Check sheet for the modelled part. Datum: model origin and axes. Units: mm. A direction names the side the tool comes from. Round coordinates to 2 decimals unless told otherwise and drop trailing zeros. Order: outer loops, then holes, each group sorted by start corner. A loop starts at its lowest first (then second) coordinate and runs counter-clockwise, first axis right, second up. Notation, with made-up numbers: (-15.5, 86.5) -> (-3.5, 86.5) arc R32 cw to (-3.5, 122.5) -> close; hole circle Ø7 at (87, 38.5). An arc over 180 degrees is marked (long way). Answer in a Markdown table with one row per item. Add a question column.
1. Material ranges on L1, parallel to X at y = 1.4, z = -2.55; L2, parallel to X at y = 2.25, z = 22.5; L3, parallel to X at y = 4.25, z = 13, recorded low to high. Write a range as from..to.
2. Draft check along Y on faces 5 (the cylindrical face through (3.55, 3.4, -2.97)), 6 (the conical face through (9.104, 5.907, 0.588)), 7 (the flat face through (9, 1.4, 2)). Enter one of: +Y half, -Y half, draft (parallel to the pull), parting line (faces both ways), or undercut.
3. Access from +Z, -Z, +X, -X, +Y, -Y to the whole of each face (thin tool, end or side, straight path). Record for faces 1 (the flat face through (16, 1.4, 17)), 2 (the flat face through (-3, 3, 4)), 3 (the cylindrical face through (-0.41, 4.9, 10.43)), 4 (the flat face through (3.9, 2.4, -1)).
4. Sectioned sample at C-C, the plane x = 3. Record the boundary of the cut face in (y, z).
5. Sectioned sample at D-D, the plane x = -2. Record the boundary of the cut face in (y, z), then the cut area to 3 significant figures.
6. Sectioned sample at B-B, the plane y = 4.75. Record the boundary of the cut face in (x, z).
7. Sectioned sample at A-A, the plane z = 11.5. Record the boundary of the cut face in (x, y).
8. Depth check by flat-ended pin: P1, Ø4.5, axis at x = 9, z = 0.26, coming from the +Y side; P2, Ø5, axis at x = 3.5, z = 23, coming from the -Y side; P3, Ø1.3, axis at x = 7.5, y = 4.5, coming from the -Z side; P4, Ø4, axis at y = 6, z = 10, coming from the -X side. Enter the tip coordinate at first touch or a pass-through.
Autodesk Inventor part; units mm, degrees
ref_plane "YZ Plane" through (0, 0, 0) normal (1, 0, 0) x (0, 1, 0)
ref_plane "XZ Plane" through (0, 0, 0) normal (0, 1, 0) x (-1, 0, 0)
ref_plane "XY Plane" through (0, 0, 0) normal (0, 0, 1) x (1, 0, 0)
sketch "Skizze1" plane through (0, 0, 0) normal (0, 1, 0) x (-1, 0, 0)
  line L0 (0, 0) -> (-18, 0)
  line L1 (-18, 0) -> (-18, 28)
  line L2 (-18, 28) -> (0, 28)
  line L3 (0, 28) -> (0, 0)
  dimension "d0" = 18
  dimension "d1" = 28
extrude "Extrusion1" add sketch "Skizze1" along normal blind 7
sketch "Skizze2" plane through (18, 0, 28) normal (0, -1, 0) x (0, 0, -1)
  line L0 (0, -18) -> (0, 0)
  line L1 (28, -18) -> (0, -18)
  line L2 (28, 0) -> (28, -18)
  line L3 (0, 0) -> (28, 0)
  line L4 (26.75, -17.25) -> (1.25, -17.25)
  line L5 (1.25, -17.25) -> (1.25, -0.75)
  line L6 (1.25, -0.75) -> (26.75, -0.75)
  line L7 (26.75, -0.75) -> (26.75, -17.25)
  line L8 (26.75, -17.25) -> (1.25, -0.75) construction
  line L9 (1.25, -17.25) -> (26.75, -0.75) construction
  point P0 (14, -9)
  dimension "d16" = 25.5
  dimension "d17" = 16.5
extrude "Extrusion2" cut sketch "Skizze2" against normal blind 1.4 contours L4 L5 L6 L7
sketch "Skizze5" plane through (18, 1.4, 28) normal (0, -1, 0) x (1, 0, 0)
  line L0 (-0.75, -1.25) -> (-0.75, -26.75)
  line L1 (-17.25, -1.25) -> (-0.75, -1.25)
  line L2 (-17.25, -26.75) -> (-17.25, -1.25)
  line L3 (-0.75, -26.75) -> (-17.25, -26.75)
  line L4 (-2.25, -25.25) -> (-2.25, -2.75)
  line L5 (-2.25, -2.75) -> (-15.75, -2.75)
  line L6 (-15.75, -2.75) -> (-15.75, -25.25)
  line L7 (-15.75, -25.25) -> (-2.25, -25.25)
  point P0 (-18, -28)
  dimension "d18" = 1.5
extrude "Extrusion5" cut sketch "Skizze5" against normal blind 6 contours L7 L6 L5 L4
ref_plane "Arbeitsebene2" through (9, 0, 0) normal (-0.7071068, 0, -0.7071068) x (0, 1, 0)
ref_plane "Arbeitsebene1" through (9, 0, 0) normal (-1, 0, 0) x (0, 0, 1)
ref_plane "Arbeitsebene3" through (0, 0, 14) normal (0, 0, 1) x (1, 0, 0)
sketch "Skizze6" plane through (0, 0, 0) normal (-1, 0, 0) x (0, 0, 1)
  line L0 (0, 7) -> (28, 7)
  line L1 (0, 0) -> (0, 7)
  line L2 (0, 0) -> (28, 0)
  line L3 (28, 0) -> (28, 7)
  line L4 (0, 7) -> (-5, 7)
  line L5 (-5, 7) -> (-5, 0)
  line L6 (-5, 0) -> (0, 0)
  line L7 (0, 0) -> (0, 7)
  dimension "d24" = 5
extrude "Extrusion6" add sketch "Skizze6" against normal up to surface (18 mm away) contours L1 L6 L5 L4
ref_plane "Arbeitsebene4" through (-15.85, 34.426, 14.0849) normal (0, 0.7071068, -0.7071068) x (1, 0, 0)
sketch "Skizze7" plane through (-15.85, 34.426, 14.0849) normal (0, 0.7071068, -0.7071068) x (1, 0, 0)
  point P0 (15.85, 34.3024)
sketch "Skizze8" plane through (0, 0, 0) normal (0, -1, 0) x (1, 0, 0)
  line L0 (0.75, 26.75) -> (17.25, 26.75)
  line L1 (17.25, 26.75) -> (17.25, 1.25)
  line L2 (17.25, 1.25) -> (0.75, 1.25)
  line L3 (0.75, 1.25) -> (0.75, 26.75)
  line L4 (0, 28) -> (18, 28)
  line L5 (18, 28) -> (18, -5)
  line L6 (0, -5) -> (0, 28)
  line L7 (0, -5) -> (-3, -5)
  line L8 (-3, -5) -> (-3, 28)
  line L9 (-3, 28) -> (0, 28)
  line L10 (0, 28) -> (0, -5)
  line L11 (18, 28) -> (18, -5)
  line L12 (18, 28) -> (21, 28)
  line L13 (21, 28) -> (21, -5)
  line L14 (21, -5) -> (18, -5)
  line L15 (18, -5) -> (18, 28)
  line L16 (0, -5) -> (0, 28)
  line L17 (0, -5) -> (18, -5)
  point P0 (0, 0)
  dimension "d27" = 3
  dimension "d28" = 3
extrude "Extrusion7" add sketch "Skizze8" against normal blind 7 contours L6 L7 L8 L9 | L12 L13 L14 L5
ref_plane "Arbeitsebene5" through (21, -5.7279, 12.7279) normal (0, 0.7071068, -0.7071068) x (-1, 0, 0)
sketch "Skizze10" plane through (-3, 0, -5) normal (-1, 0, 0) x (0, 0, 1)
  line L0 (0, 7) -> (33, 7)
  line L1 (0, 0) -> (0, 7)
  line L2 (33, 0) -> (0, 0)
  line L3 (33, 0) -> (33, 7)
  circle A0 centre (16.5, 3.9193) radius 1.45
  point P0 (5, 0)
  dimension "d38" = 2.9
extrude "Extrusion9" cut sketch "Skizze10" against normal through all contours A0
ref_plane "Arbeitsebene6" through (21, -1.4853, 8.4853) normal (0, 0.7071068, -0.7071068) x (-1, 0, 0)
sketch "Skizze14" plane through (21, 0, -5) normal (0, 0, -1) x (-1, 0, 0)
  line L0 (24, 0) -> (0, 0)
  line L1 (3.75, 1.4) -> (20.25, 1.4)
  circle A0 centre (17.5107, 1.4) radius 0.9
  circle A1 centre (7.1764, 1.4) radius 1.0097
  point P0 (21, 0)
  dimension "d55" = 1.8
hole "Bohrung3" at (3.4893, 1.4, -5) at (13.8236, 1.4, -5) direction (0, 0, 1) diameter 1.8 depth 10 tip angle 118 counterbore diameter 4 counterbore depth 4
sketch "Skizze15" plane through (21, 0, 28) normal (1, 0, 0) x (0, 0, -1)
  circle A0 centre (16.5, 3.9193) radius 1.45
  line L0 (0, 7) -> (33, 7)
  line L1 (0, 0) -> (0, 7)
  line L2 (33, 0) -> (0, 0)
  line L3 (33, 0) -> (33, 7)
  line L4 (25.25, 7) -> (5, 7)
  line L5 (10.6096, 7) -> (10.6096, 0)
  point P0 (28, 0)
extrude "Extrusion10" add sketch "Skizze15" along normal blind 4 contours L0 L5 L2 L1
sketch "Skizze16" plane through (-3, 0, -5) normal (-1, 0, 0) x (0, 0, 1)
  line L0 (33, 7) -> (33, 0)
  line L1 (33, 0) -> (22.3904, 0)
  line L2 (22.3904, 0) -> (22.3904, 7)
  line L3 (22.3904, 7) -> (33, 7)
  point P0 (5, 0)
extrude "Extrusion11" add sketch "Skizze16" along normal blind 4
sketch "Skizze13" plane through (21, 7, 8.4853) normal (0, 1, 0) x (-1, 0, 0)
  circle A0 centre (-2, 12.7713) radius 2.45
  circle A1 centre (26, 12.7713) radius 2.45
  circle A2 centre (12, -8.2287) radius 2.75
  point P0 (21, -4.9497)
  point P1 (12, -10.2287)
hole "Bohrung2" at (23, 7, 21.2566) at (-5, 7, 21.2566) at (9, 7, 0.2566) direction (0, -1, 0) diameter 4 depth 0.1 tip angle 118
chamfer "Fase3" distance 4 angle 45 4 edges at (21, 3.5, 17.3904) (-3, 3.5, 17.3904) (9, 7, 28) (9, 7, -5)
properties part number "20_Cube_Insert_Fibercombiner_FPC_filtermount_v3"
Answer key:
| question | item | result |
|---|---|---|
| 1 | L1 | x = -3..1.49, 5.49..11.82, 15.82..21 |
| 1 | L2 | x = -7..2.25, 15.75..25 |
| 1 | L3 | x = -3..2.25, 15.75..21 |
| 2 | face 5 | undercut |
| 2 | face 6 | +Y half |
| 2 | face 7 | -Y half |
| 3 | face 1 | -Y |
| 3 | face 2 | -Z, -X, +Y, -Y |
| 3 | face 3 | +X, -X |
| 3 | face 4 | -Z |
| 4 | outline | (0, -1) -> (0.64, -1) -> (0.64, 1.25) -> (0, 1.25) -> close; (0, 26.75) -> (1.4, 26.75) -> (1.4, 25.25) -> (5.75, 25.25) -> (3, 28) -> (0, 28) -> close; (2.16, -1) -> (3.34, -1) -> (3.34, -4.66) -> (7, -1) -> (7, 2.75) -> (2.16, 2.75) -> close |
| 5 | outline | (0, -5) -> (3, -5) -> (7, -1) -> (7, 24) -> (3, 28) -> (0, 28) -> close; hole circle Ø2.9 at (3.92, 11.5) |
| 5 | area | 208 mm² |
| 6 | outline | (-7, 17.39) -> (-3, 13.39) -> (-3, 12.69) -> (2.25, 12.69) -> (2.25, 25.25) -> (15.75, 25.25) -> (15.75, 12.69) -> (21, 12.69) -> (21, 13.39) -> (25, 17.39) -> (25, 26.25) -> (-7, 26.25) -> close; (-3, -3.25) -> (21, -3.25) -> (21, 10.31) -> (15.75, 10.31) -> (15.75, 2.75) -> (2.25, 2.75) -> (2.25, 10.31) -> (-3, 10.31) -> close |
| 7 | outline | (-3, 0) -> (0.75, 0) -> (0.75, 1.4) -> (2.25, 1.4) -> (2.25, 2.47) -> (-3, 2.47) -> close; (-3, 5.37) -> (2.25, 5.37) -> (2.25, 7) -> (-3, 7) -> close; (15.75, 1.4) -> (17.25, 1.4) -> (17.25, 0) -> (21, 0) -> (21, 2.47) -> (15.75, 2.47) -> close; (15.75, 5.37) -> (21, 5.37) -> (21, 7) -> (15.75, 7) -> close |
| 8 | P1 | stops at y = 7 |
| 8 | P2 | stops at y = 1.4 |
| 8 | P3 | stops at z = -4.15 |
| 8 | P4 | stops at x = -3 |
